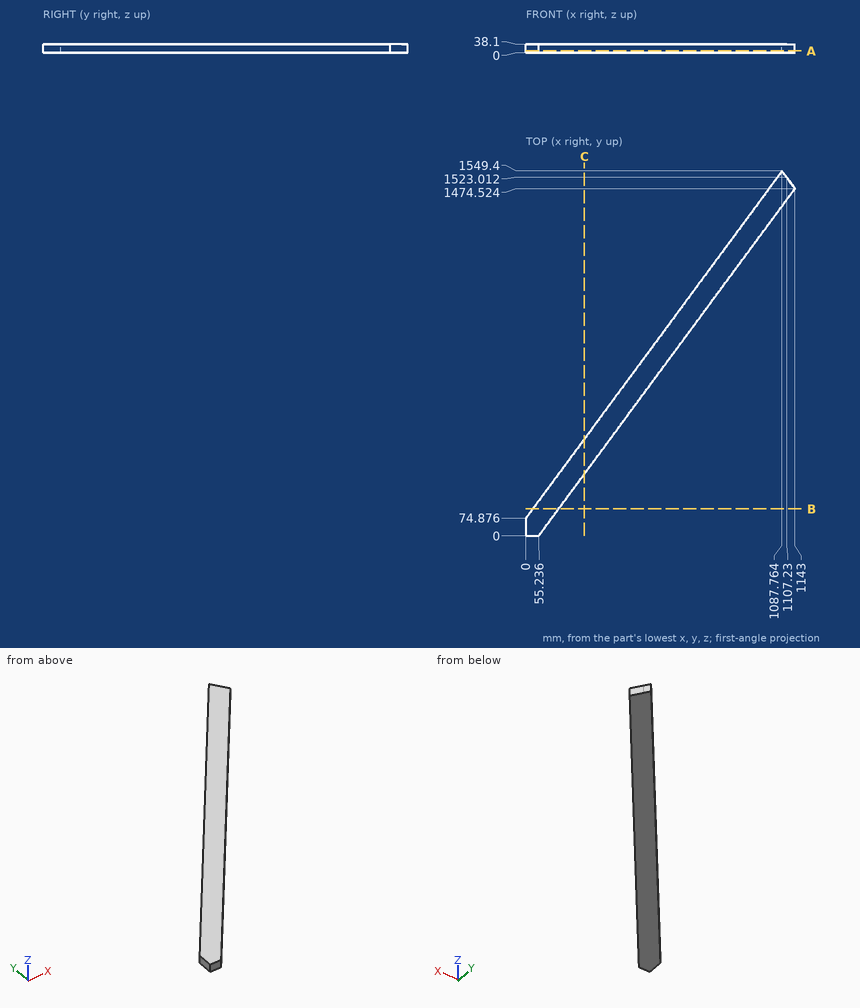
Could you check a few things on this drawing? It's one solid part, dimensions in mm from its lowest x, y, z. Round coordinates to 2 decimals unless told otherwise and drop trailing zeros. Write each loop counter-clockwise with the first axis right and the second up, starting at its lowest first coordinate (ties: lowest second). Pieces come first, ordered by that corner, then holes. Notation, with made-up numbers: (83.5, -30.5) -> (110.5, -30.5) arc R10 ccw to (110.5, -17.5) -> close; hole circle Ø6 at (72, -26). An arc over 180 degrees is marked (long way). Use one line per item in the form item = value. Start each with the question number.
Q1. Imagine slicing it at B-B (y = 114). Please give me the cut outline in (x, z) (1 decimal).
Q2. Imagine slicing it at C-C (x = 248). Please give me the cut outline in (y, z), then the cut area to 3 significant figures.
Q3. I'm going to push flat-ended pins straight in: P1, Ø1, axis at x = 902.5, z = 32, coming from the -Y side (1 decimal); P2, Ø4, axis at x = 579, z = 34, coming from the -Y side; P3, Ø5, axis at y = 377, z = 26.5, coming from the -X side (1 decimal). Where does each tip first touch, or does it pass through?
Q4. Imagine slicing it at A-A (z = 9). Please give me the cut outline in (x, y), then the cut area to 3 significant figures.
Q5. If I drill on probe 1 along X at (y, z) = (717, 7.5); probe 2 along X at (y, z) = (185, 35); probe 3 along Y at (x, z) = (490, 27) (1 decimal), over which ranges is the centre line in solid material (lowest first)? Write a range as [from, to].
Worked out:
q1.outline = (28.9, 0) -> (139.3, 0) -> (139.3, 38.1) -> (28.9, 38.1) -> close
q2.outline = (261.3, 0) -> (411.05, 0) -> (411.05, 38.1) -> (261.3, 38.1) -> close
q2.area = 5,710 mm^2
q3.P1 = 1147.8
q3.P2 = 707.28
q3.P3 = 221
q4.outline = (0, 0) -> (55.24, 0) -> (1143, 1474.52) -> (1107.23, 1523.01) -> (1087.76, 1549.4) -> (0, 74.88) -> close
q4.area = 165,000 mm^2
q5.probe_1 = [473.7, 584.17]
q5.probe_2 = [81.24, 191.71]
q5.probe_3 = [589.3, 739.1]
